Check sheet for the modelled part. Datum: model origin and axes. Units: mm. A direction names the side the tool comes from. Give positions to 0.01 mm unless a question says otherwise; leave off trailing zeros. Order: outer loops, then holes, each group sorted by start corner. A loop starts at its lowest first (then second) coordinate and runs counter-clockwise, first axis right, second up.
from build123d import *

# Parameters (mm, degrees)
F2_W          = 56.6284824163
F2_H          = 136.3001726568
F3_DEPTH      = 25.4
F0_R          = 38.1
F4_DEPTH      = 25.4
F1_R          = 38.1
F5_DEPTH      = 25.4
F6_D          = 50.8
F8_D          = 50.8
F11_T4_DEPTH  = 25.4
F11_S5_R      = 25.4
F11_T6_DEPTH  = 43
F11_T10_DEPTH = 25.4
F11_S11_R     = 25.4
F11_T12_DEPTH = 43
F11_T16_DEPTH = 25.4
F11_S17_R     = 25.4
F11_T18_DEPTH = 43
F11_T22_DEPTH = 25.4
F11_S23_R     = 25.4
F11_T24_DEPTH = 43


# Not quite as in the source:
# - a fillet or chamfer that OpenCascade refuses, or shapes differently, is made with other operations: its cross-section is extruded or revolved along the edge and cut away or added
# - two fillets or chamfers of one size are made in one step


with BuildPart() as f3:
    # F2 (on Right) → F3 (new body)
    with BuildSketch(Plane.YZ):
        with Locations((-0.1386040822, -92.7020926028)):
            Rectangle(F2_W, F2_H)
    extrude(amount=F3_DEPTH)

    # F0 (on Right) → F4 (join)
    with BuildSketch(Plane.YZ):
        Circle(F0_R)
    extrude(amount=F4_DEPTH)

    # F1 (on Right) → F5 (join)
    with BuildSketch(Plane.YZ):
        with Locations((0, -185.5300813913)):
            Circle(F1_R)
    extrude(amount=F5_DEPTH)

    # F6 (through all)
    with Locations(Plane(origin=(0, 0, 0), x_dir=(0, 1, 0), z_dir=(-1, 0, 0))):
        with Locations((0, 0)):
            Hole(F6_D / 2)

    # F8 (through all)
    with Locations(Plane.YZ.offset(25.4)):
        with Locations((0, -185.5300813913)):
            Hole(F8_D / 2)

    # F11: fillet of radius 254 on 4 edges, made by hand


with BuildPart() as f11_tool2:
    # F11_s3 → F11_t4 (new body)
    with BuildSketch(Plane.YZ.offset(25.4)):
        with BuildLine():
            add(Edge.make_bspline(
                [(-28.4524452903, -111.0798377649), (-28.4524452903, -143.9931007722), (-36.841297299, -175.8193484896)],
                knots=[0, 0, 0, 1, 1, 1], degree=2, weights=[1, 1, 1]))
            Line((-36.841297299, -175.8193484896), (-12.2799424998, -182.293299562))
            ThreePointArc((-12.2799424998, -182.293299562), (-11.1895620368, -179.5236177494), (-9.4841025329, -177.0840347894))
            Line((-9.4841025329, -177.0840347894), (-3.0526052903, -160.1914627454))
            ThreePointArc((-3.0526052903, -160.1914627454), (-3.0526052903, -135.6356502551), (-3.0522052903, -111.0798377649))
            Line((-3.0522052903, -111.0798377649), (-28.4524452903, -111.0798377649))
        make_face()
    extrude(amount=-F11_T4_DEPTH)

    # F11_s5 → F11_t6 (cut, symmetric)
    with BuildSketch(Plane.YZ.offset(12.7)):
        with Locations((0, -185.5300813913)):
            Circle(F11_S5_R)
    extrude(amount=F11_T6_DEPTH, both=True, mode=Mode.SUBTRACT)


with BuildPart() as f3_1:
    add(f3.part)

    # F11_t1: union F11_tool2
    add(f11_tool2.part)


with BuildPart() as f11_tool8:
    # F11_s9 → F11_t10 (new body)
    with BuildSketch(Plane.YZ.offset(25.4)):
        with BuildLine():
            add(Edge.make_bspline(
                [(-36.841297299, -9.7107329018), (-28.4524452903, -41.5369806191), (-28.4524452903, -74.4502436264)],
                knots=[0, 0, 0, 1, 1, 1], degree=2, weights=[1, 1, 1]))
            Line((-28.4524452903, -74.4502436264), (-3.0522052903, -74.4502436264))
            ThreePointArc((-3.0522052903, -74.4502436264), (-3.0526052903, -49.8944311362), (-3.0526052903, -25.338618646))
            Line((-3.0526052903, -25.338618646), (-9.4841025329, -8.446046602))
            ThreePointArc((-9.4841025329, -8.446046602), (-11.1895620368, -6.0064636419), (-12.2799424998, -3.2367818293))
            Line((-12.2799424998, -3.2367818293), (-36.841297299, -9.7107329018))
        make_face()
    extrude(amount=-F11_T10_DEPTH)

    # F11_s11 → F11_t12 (cut, symmetric)
    with BuildSketch(Plane.YZ.offset(12.7)):
        Circle(F11_S11_R)
    extrude(amount=F11_T12_DEPTH, both=True, mode=Mode.SUBTRACT)


with BuildPart() as f3_2:
    add(f3_1.part)

    # F11_t7: union F11_tool8
    add(f11_tool8.part)


with BuildPart() as f11_tool14:
    # F11_s15 → F11_t16 (new body)
    with BuildSketch(Plane.YZ.offset(25.4)):
        with BuildLine():
            add(Edge.make_bspline(
                [(36.8051403395, -9.8468860434), (28.175237126, -42.1032559751), (28.175237126, -75.4941024849)],
                knots=[0, 0, 0, 1, 1, 1], degree=2, weights=[1, 1, 1]))
            Line((28.175237126, -75.4941024849), (2.774997126, -75.4941024849))
            ThreePointArc((2.774997126, -75.4941024849), (2.775397126, -50.5703062168), (2.775397126, -25.6465099486))
            Line((2.775397126, -25.6465099486), (9.3917015577, -8.5486750967))
            ThreePointArc((9.3917015577, -8.5486750967), (11.1455038849, -6.0878277907), (12.2678906608, -3.2821643992))
            Line((12.2678906608, -3.2821643992), (36.8051403395, -9.8468860434))
        make_face()
    extrude(amount=-F11_T16_DEPTH)

    # F11_s17 → F11_t18 (cut, symmetric)
    with BuildSketch(Plane.YZ.offset(12.7)):
        Circle(F11_S17_R)
    extrude(amount=F11_T18_DEPTH, both=True, mode=Mode.SUBTRACT)


with BuildPart() as f3_3:
    add(f3_2.part)

    # F11_t13: union F11_tool14
    add(f11_tool14.part)


with BuildPart() as f11_tool20:
    # F11_s21 → F11_t22 (new body)
    with BuildSketch(Plane.YZ.offset(25.4)):
        with BuildLine():
            add(Edge.make_bspline(
                [(28.175237126, -110.0359789064), (28.175237126, -143.4268254163), (36.8051403395, -175.683195348)],
                knots=[0, 0, 0, 1, 1, 1], degree=2, weights=[1, 1, 1]))
            Line((36.8051403395, -175.683195348), (12.2678906608, -182.2479169921))
            ThreePointArc((12.2678906608, -182.2479169921), (11.1455038849, -179.4422536006), (9.3917015577, -176.9814062946))
            Line((9.3917015577, -176.9814062946), (2.775397126, -159.8835714427))
            ThreePointArc((2.775397126, -159.8835714427), (2.775397126, -134.9597751745), (2.774997126, -110.0359789064))
            Line((2.774997126, -110.0359789064), (28.175237126, -110.0359789064))
        make_face()
    extrude(amount=-F11_T22_DEPTH)

    # F11_s23 → F11_t24 (cut, symmetric)
    with BuildSketch(Plane.YZ.offset(12.7)):
        with Locations((0, -185.5300813913)):
            Circle(F11_S23_R)
    extrude(amount=F11_T24_DEPTH, both=True, mode=Mode.SUBTRACT)


with BuildPart() as f3_4:
    add(f3_3.part)

    # F11_t19: union F11_tool20
    add(f11_tool20.part)


solid = f3_4.part
1) Section check A-A, the plane z = 0. Record the cut outline in (x, y), then the cut area to 3 significant figures.
Recorded:
outline: (0, -38.1) - (25.4, -38.1) - (25.4, -25.4) - (0, -25.4) - close; (0, 25.4) - (25.4, 25.4) - (25.4, 38.1) - (0, 38.1) - close
area: 645 mm2
2) Material ranges on L1, parallel to Z at x = 5.75, y = 0; L2, parallel to Z at x = 15.25, y = 2; L3, parallel to Y at x = 6, z = -19, recorded low to high.
Recorded:
L1: z = -223.63 to -210.93, -160.13 to -25.4, 25.4 to 38.1
L2: z = -223.58 to -210.85, -160.21 to -25.32, 25.32 to 38.05
L3: y = -34.58 to -16.86, 16.86 to 34.54
3) Section check C-C, the plane x = 15.25. State how many separate pieces and enclosed holes the cut face has, then the cut area to 3 significant figures.
Recorded:
separate pieces: 1
enclosed holes: 2
area: 12,100 mm2
4) Set-up check for faces 1 (the face through (12.878, -11.721, 22.534)), 2 (the face through (13, 28.176, -93)): record each of +Z, -Z, +X, -X, +Y, -Y from which the full face is reachable in a straight line by a thin tool's end or side.
Recorded:
face 1: +X, -X
face 2: +X, -X, +Y
5) Section check B-B, the plane y = 0. Record the cut outline in (x, z).
Recorded:
outline: (0, -223.63) - (25.4, -223.63) - (25.4, -210.93) - (0, -210.93) - close; (0, -160.13) - (25.4, -160.13) - (25.4, -25.4) - (0, -25.4) - close; (0, 25.4) - (25.4, 25.4) - (25.4, 38.1) - (0, 38.1) - close
6) Draft check along Z on faces 3 (the face through (13, -28.453, -93)), 4 (the face through (0, -1, -91)). Enter one of: +Z half, -Z half, draft (parallel to the pull), parting line (faces both ways), or undercut.
Recorded:
face 3: undercut
face 4: draft
7) Section check D-D, the plane y = 19.5. Record the cut outline in (x, z).
Recorded:
outline: (0, -218.26) - (25.4, -218.26) - (25.4, -201.81) - (0, -201.81) - close; (0, -169.25) - (25.4, -169.25) - (25.4, -16.28) - (0, -16.28) - close; (0, 16.28) - (25.4, 16.28) - (25.4, 32.73) - (0, 32.73) - close
8) Depth check by flat-ended pin: pin 1 Ø6 at (x, z) = (14.5, -136.5) entering from +Y; pin 2 Ø10 at (x, y) = (6.5, 16) entering from -Z; pin 3 Ø8 at (x, y) = (5.5, -20.5) entering from +Z. Enter the tip coordinate at first touch or a pass-through.
Recorded:
pin 1: stops at y = 29.88
pin 2: stops at z = -222.01
pin 3: stops at z = 34.34
